Read the model definition and answer for the solid it produces. Units are mm, in the model's axes. Face numbers are marked on the shaded views. Round coordinates to 2 decimals unless told otherwise and drop trailing zeros. Write each loop counter-clockwise with the first axis right and the second up, starting at its lowest first coordinate (ties: lowest second). Pieces come first, ordered by that corner, then holes. Notation, with made-up numbers: (75, -16) - (133, -16) arc R23 ccw to (133, 14) - close; hole circle Ø6 at (12, 4). An arc over 180 degrees is marked (long way). Use one line per item in the form item = value. Start each with the question number.
1) The part is cut by section D-D, the plane x = 0. Give the vertices of the cut face in (y, z).
2) The part is cut by section C-C, the plane y = 284. Give the vertices of the cut face in (x, z), plus the area to 3 significant figures.
3) Consider line 1 along X through (y, z) = (337.75, 0); line 2 along X through (y, z) = (335.5, 0); line 3 along Y through (x, z) = (0, -5). Determine where each line is inside the solid, lowest interval first. Write a range as from..to.
4) The part is cut by section A-A, the plane y = 75. Give the vertices of the cut face in (x, z), plus the area to 3 significant figures.
5) For a pull along X with two mould halves and no side action, classify the marked faces 1, 2 and 3 as released by +X, released by -X, zero draft, split by the parting line, or undercut.
6) The part is cut by section B-B, the plane x = -120. Give the vertices of the cut face in (y, z).
7) Each of these flat-tipped pins is pushed along its axis until it touches: pin 1 (3 mm diameter, centred on x = -72.5, z = 3, fed in from +Y); pin 2 (1 mm diameter, centred on x = -98.5, y = 106, fed in from +Z). Where does it stop, or does it pass through?
from build123d import *

# Parameters (mm, degrees)
SKETCH1_W                    = 280
SKETCH1_H                    = 30
BOSS_EXTRUDE1_DEPTH          = 350
CUT_EXTRUDE1_DEPTH           = 350
CHAMFER1_SIZE                = 70
M10_TAPPED_HOLE3_D           = 8.5
M10_TAPPED_HOLE3_DEPTH       = 24.5
M10_TAPPED_HOLE3_CSINK_D     = 10.05
M10_TAPPED_HOLE3_CSINK_ANGLE = 90
M10_TAPPED_HOLE3_TIP         = 2.553657631
SKETCH11_R                   = 8.75
CUT_EXTRUDE3_DEPTH           = 350
SKETCH12_R                   = 15
CUT_EXTRUDE4_DEPTH           = 350
SKETCH13_R                   = 31
CUT_EXTRUDE5_DEPTH           = 16


with BuildPart() as part:
    # Sketch1 → Boss-Extrude1 (new body)
    with BuildSketch(Plane(origin=(0, 0, 0), x_dir=(1, 0, 0), z_dir=(0, 1, 0))):
        Rectangle(SKETCH1_W, SKETCH1_H)
    extrude(amount=BOSS_EXTRUDE1_DEPTH)

    # Sketch2 → Cut-Extrude1 (cut)
    with BuildSketch(Plane.XY.offset(15)):
        with BuildLine():
            Line((50, 350), (50, 175))
            ThreePointArc((50, 175), (0, 125), (-50, 175))
            Line((-50, 175), (-50, 350))
            ThreePointArc((-50, 350), (0, 400), (50, 350))
        make_face()
    extrude(amount=-CUT_EXTRUDE1_DEPTH, mode=Mode.SUBTRACT)

    # Chamfer1
    chamfer1_edges = [part.edges().sort_by_distance(p)[0] for p in [
        (-140, 350, 0),
        (140, 350, 0),
    ]]
    chamfer(chamfer1_edges, length=CHAMFER1_SIZE)

    # M10 Tapped Hole3
    with Locations(Plane(origin=(-60, 350, 0), x_dir=(0, 0, 1), z_dir=(0, 1, 0))):
        with Locations((0, 0), (0, 120)):
            CounterSinkHole(M10_TAPPED_HOLE3_D / 2, M10_TAPPED_HOLE3_CSINK_D / 2, depth=M10_TAPPED_HOLE3_DEPTH, counter_sink_angle=M10_TAPPED_HOLE3_CSINK_ANGLE)
            with Locations((0, 0, -(M10_TAPPED_HOLE3_DEPTH + M10_TAPPED_HOLE3_TIP / 2))):  # 118° drill point
                Cone(0, M10_TAPPED_HOLE3_D / 2, M10_TAPPED_HOLE3_TIP, mode=Mode.SUBTRACT)

    # Sketch11 → Cut-Extrude3 (cut)
    with BuildSketch(Plane.XY.offset(15)):
        with Locations((-120, 55)):
            Circle(SKETCH11_R)
        with Locations((120, 55)):
            Circle(SKETCH11_R)
    extrude(amount=-CUT_EXTRUDE3_DEPTH, mode=Mode.SUBTRACT)

    # Sketch12 → Cut-Extrude4 (cut)
    with BuildSketch(Plane.XY.offset(15)):
        with Locations((-75, 124.749371855)):
            Circle(SKETCH12_R)
        with Locations((75, 124.749371855)):
            Circle(SKETCH12_R)
        with Locations((0, 75)):
            Circle(SKETCH12_R)
    extrude(amount=-CUT_EXTRUDE4_DEPTH, mode=Mode.SUBTRACT)

    # Sketch13 → Cut-Extrude5 (cut)
    with BuildSketch(Plane.XY.offset(15)):
        with Locations((-75, 124.749371855)):
            Circle(SKETCH13_R)
        with Locations((0, 75)):
            Circle(SKETCH13_R)
        with Locations((75, 124.749371855)):
            Circle(SKETCH13_R)
    extrude(amount=-CUT_EXTRUDE5_DEPTH, mode=Mode.SUBTRACT)


solid = part.part
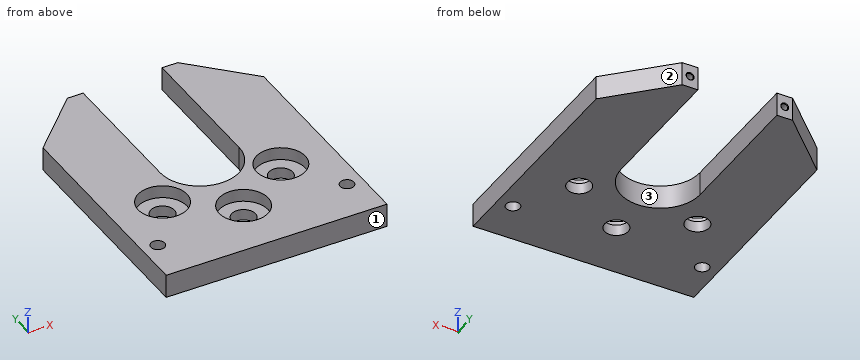
Geometry results:
q1.outline = (0, -15) - (60, -15) - (60, -1) - (44, -1) - (44, 15) - (0, 15) - close; (90, -15) - (125, -15) - (125, 15) - (106, 15) - (106, -1) - (90, -1) - close
q2.outline = (-136, -15) - (-50, -15) - (-50, 15) - (-136, 15) - close; (50, -15) - (136, -15) - (136, 15) - (50, 15) - close
q2.area = 5,160 mm2
q3.line_1 = -82.25..-64.25, -55.75..-50, 50..55.75, 64.25..82.25
q3.line_2 = -84.5..-64.25, -55.75..-50, 50..55.75, 64.25..84.5
q3.line_3 = 0..60, 90..125
q4.outline = (-140, -15) - (-15, -15) - (-15, -1) - (-31, -1) - (-31, 15) - (-140, 15) - close; (15, -15) - (140, -15) - (140, 15) - (31, 15) - (31, -1) - (15, -1) - close
q4.area = 6,990 mm2
q5.face_1 = zero draft
q5.face_2 = released by +X
q5.face_3 = undercut
q6.outline = (0, -15) - (46.25, -15) - (46.25, 15) - (0, 15) - close; (63.75, -15) - (300, -15) - (300, 15) - (63.75, 15) - close
q7.pin_1 = 349
q7.pin_2 = -1
